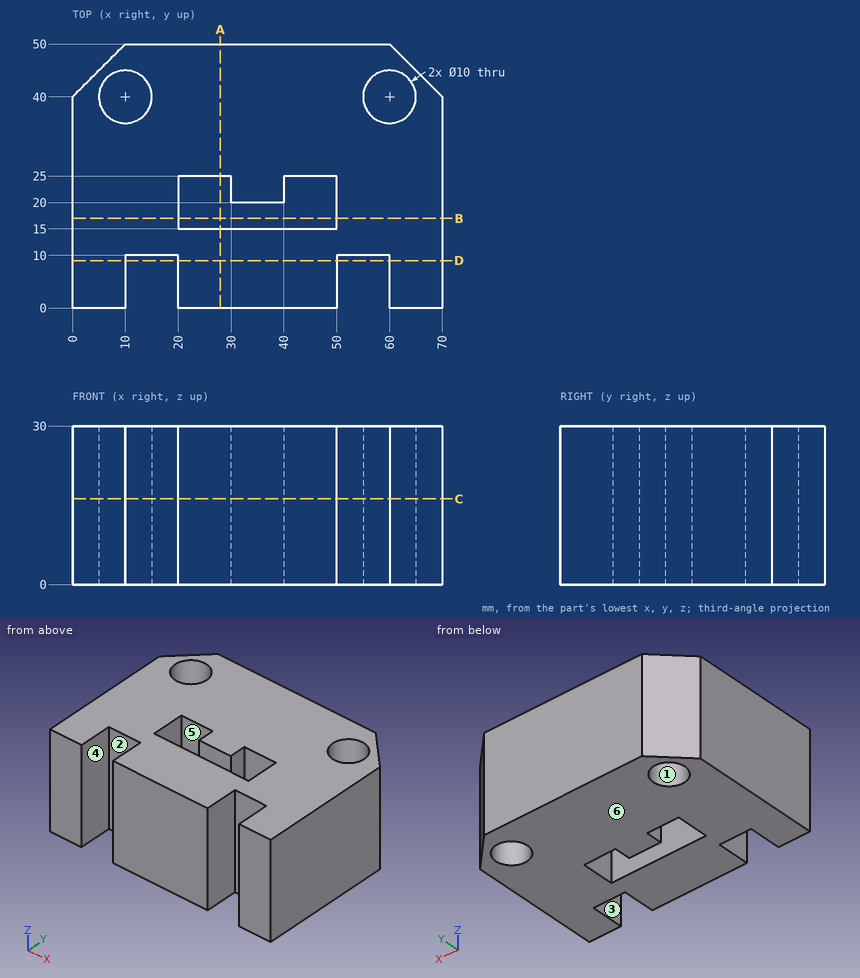
For this review, use the dimensioned drawing (mm, ordinates from the lowest corner) and the shaded views. A direction names the side the tool comes from. Give positions to 0.01 mm unless a question says otherwise; leave off trailing zeros. Order: outer loops, then holes, each group sorted by start corner. A loop starts at its lowest first (then second) coordinate and runs counter-clockwise, first axis right, second up.
1. Add section D-D, the plane y = 9. State the section outline as (x, z) points, then the cut area to 3 significant figures.
Solution:
outline: (0, 0) - (10, 0) - (10, 30) - (0, 30) - close; (20, 0) - (50, 0) - (50, 30) - (20, 30) - close; (60, 0) - (70, 0) - (70, 30) - (60, 30) - close
area: 1,500 mm2
2. To check wall thickness, follow L1, parallel to Y at x = 42, z = 4; L2, parallel to Y at x = 37, z = 10; L3, parallel to X at y = 38, z = 10.25. State the ranges of each line that lie inside material, in increasing order.
Solution:
L1: y = 0 to 15, 25 to 50
L2: y = 0 to 15, 20 to 50
L3: x = 0 to 5.42, 14.58 to 55.42, 64.58 to 70
3. For pin 1 Ø5 at (y, z) = (27, 9.5) entering from -X; pin 2 Ø8 at (x, z) = (15, 11.5) entering from -Y; pin 3 Ø6 at (x, y) = (60, 40) entering from +Z, all flat-tipped, find the tip position at first contact; note any pin that passes through.
Solution:
pin 1: stops at x = 0
pin 2: stops at y = 10
pin 3: passes through
4. Tool access review of the marked faces 4, 5 and 6: name each direction out of +Z, -Z, +X, -X, +Y, -Y from which nothing blocks a thin tool from reaching the whole face with its end or side.
Solution:
face 4: +Z, -Z, -Y
face 5: +Z, -Z
face 6: -Z, +X, -X, +Y, -Y
5. Add section C-C, the plane z = 16.25. State the section outline as (x, y) points, then the cut area to 3 significant figures.
Solution:
outline: (0, 0) - (10, 0) - (10, 10) - (20, 10) - (20, 0) - (50, 0) - (50, 10) - (60, 10) - (60, 0) - (70, 0) - (70, 40) - (60, 50) - (10, 50) - (0, 40) - close; hole circle Ø10 at (10, 40); hole (20, 15) - (50, 15) - (50, 25) - (40, 25) - (40, 20) - (30, 20) - (30, 25) - (20, 25) - close; hole circle Ø10 at (60, 40)
area: 2,790 mm2
6. Add section B-B, the plane y = 17. State the section outline as (x, z) points, then the cut area to 3 significant figures.
Solution:
outline: (0, 0) - (20, 0) - (20, 30) - (0, 30) - close; (50, 0) - (70, 0) - (70, 30) - (50, 30) - close
area: 1,200 mm2
7. Mouldability with a two-part tool opening along Y and no side actions: class the marked faces 1, 2 and 3 as +Y half, -Y half, draft (parallel to the pull), parting line (faces both ways), or undercut.
Solution:
face 1: undercut
face 2: -Y half
face 3: draft
8. Add section A-A, the plane x = 28. State the section outline as (y, z) points.
Solution:
outline: (0, 0) - (15, 0) - (15, 30) - (0, 30) - close; (25, 0) - (50, 0) - (50, 30) - (25, 30) - close
